Design review of the part built by this model. Coordinates are the model's own, in mm. A direction names the side the tool comes from. Coordinates: 2 decimals unless noted, no trailing zeros. Loops run counter-clockwise (first coordinate to the right, second up) from the corner with the lowest first, then second, coordinate; pieces in that order, holes last.
Q1. For P1, Ø0.5, axis at x = -14, z = 1, coming from the -Y side; P2, Ø0.8, axis at y = -2.5, z = 0.5, coming from the +X side, all flat-tipped, find the tip position at first contact; note any pin that passes through.
Q2. Add section A-A on y = 4. Give the boundary of the cut face in (x, z).
Q3. Machinability: for faces 1 (the face through (1.52, 8.87, 0.78)), 2 (the face through (-12, 4.877, 1)), 3 (the face through (9, 7, 1.588)), which of the approach directions +Z, -Z, +X, -X, +Y, -Y give a long, thin tool a straight path to every point of the face, cutting with its end or side? Answer none if there is none.
Q4. Add section B-B on x = 5.5. Give the boundary of the cut face in (y, z), and give its area (3 significant figures).
Q5. Add section C-C on z = 1.1. Give the number of separate pieces and of enclosed holes in the cut face, and give its area (3 significant figures).
Q6. Draft analysis for pull direction X (two halves, no side actions). For faces 4 (the face through (-13.07, 14, 0.78)), 5 (the face through (10.44, -1.11, 0.78)), 6 (the face through (16.226, 7.464, 0.783)), state which applies: released by +X, released by -X, zero draft, split by the parting line, or undercut.
Q7. Wall thickness on probe 1 along X at (y, z) = (12.5, 1.35); probe 2 along Y at (x, z) = (8.5, 0.3); probe 3 along X at (y, z) = (13, 1.05): over which ranges is each line inside the solid? List them lowest first.
Q8. Add section D-D on y = -15. Give the boundary of the cut face in (x, z).
```python
from build123d import *
from build123d.topology import SkipClean

# Parameters (mm, degrees)
SKETCH1_R           = 1.4224
BOSS_EXTRUDE1_DEPTH = 1.5875
CUT_EXTRUDE3_DEPTH  = 31.574112518
CUT_EXTRUDE4_DEPTH  = 31.574112518
SKETCH4_R           = 1.1049
BOSS_EXTRUDE2_DEPTH = 1.5875
SKETCH4_3_R         = 1.1049
CUT_EXTRUDE5_DEPTH  = 2.54


with BuildPart() as part:
    # Sketch1 → Boss-Extrude1 (new body)
    with BuildSketch(Plane.XY):
        with BuildLine():
            Line((-5.027565338, -0.720652536), (-4.515281158, 3.5306))
            Line((-4.515281158, 3.5306), (-2.860140414, 4.994714494))
            Line((-2.860140414, 4.994714494), (-4.980602482, 7.391837931))
            Line((-4.980602482, 7.391837931), (-2.583479045, 9.5123))
            Line((-2.583479045, 9.5123), (-0.463016976, 7.115176563))
            Line((-0.463016976, 7.115176563), (11.876076152, 18.030166811))
            ThreePointArc((11.876076152, 18.030166811), (-16.886200405, -13.453041882), (20.228041911, 7.546815251))
            Line((20.228041911, 7.546815251), (8.405899773, -2.910887338))
            Line((8.405899773, -2.910887338), (10.526361842, -5.308010776))
            Line((10.526361842, -5.308010776), (8.129238404, -7.428472845))
            Line((8.129238404, -7.428472845), (6.008776335, -5.031349407))
            Line((6.008776335, -5.031349407), (4.353635591, -6.495463901))
            Line((4.353635591, -6.495463901), (1.815981702, -6.489359631))
            Line((1.815981702, -6.489359631), (-5.455454601, -12.9215711))
            Line((-5.455454601, -12.9215711), (-8.720293025, -9.230761998))
            Line((-8.720293025, -9.230761998), (-2.425370717, -3.662361234))
            Line((-2.425370717, -3.662361234), (-5.027565338, -0.720652536))
        make_face()
        with Locations((0, 18.415)):
            Circle(SKETCH1_R, mode=Mode.SUBTRACT)
        with Locations((0, -18.415)):
            Circle(SKETCH1_R, mode=Mode.SUBTRACT)
    extrude(amount=BOSS_EXTRUDE1_DEPTH)

    # Sketch2 → Cut-Extrude3 (cut, through all)
    with BuildSketch(Plane.XY.offset(1.5875)):
        with BuildLine():
            Line((-7.084965338, 4.8768), (-21.031997569, 4.8768))
            ThreePointArc((-21.031997569, 4.8768), (-21.588987692, -0.209070373), (-20.933606898, -5.2832))
            Line((-20.933606898, -5.2832), (-7.084965338, -5.2832))
            Line((-7.084965338, -5.2832), (-7.084965338, 4.8768))
        make_face()
    extrude(amount=-CUT_EXTRUDE3_DEPTH, mode=Mode.SUBTRACT)

    # Sketch3 → Cut-Extrude4 (cut, through all)
    with BuildSketch(Plane(origin=(0, 0, 0), x_dir=(-1, 0, 0), z_dir=(0, 0, -1))):
        with BuildLine():
            Line((-20.871224203, -5.5245), (-16.984058744, -5.5245))
            Line((-16.984058744, -5.5245), (-16.984058744, 4.677232838))
            Line((-16.984058744, 4.677232838), (-20.228041911, 7.546815251))
            ThreePointArc((-20.228041911, 7.546815251), (-21.563910577, 1.061065789), (-20.871224203, -5.5245))
        make_face()
    extrude(amount=-CUT_EXTRUDE4_DEPTH, mode=Mode.SUBTRACT)

    # Sketch4 → Boss-Extrude2 (add)
    # profile 1 of 5: a face of its own
    with BuildSketch(Plane(origin=(0, 0, 0), x_dir=(-1, 0, 0), z_dir=(0, 0, -1))):
        with BuildLine():
            Line((-16.984058744, 5.5245), (-16.984058744, 4.677232838))
            Line((-16.984058744, 4.677232838), (-12.420130291, 0.640045174))
            Line((-12.420130291, 0.640045174), (-3.551213542, 10.666109075))
            Line((-3.551213542, 10.666109075), (-8.959431605, 15.450143591))
            ThreePointArc((-8.959431605, 15.450143591), (-11.076965007, 14.009967805), (-12.966760902, 12.28175327))
            Line((-12.966760902, 12.28175327), (-15.004080987, 13.83506338))
            ThreePointArc((-15.004080987, 13.83506338), (-17.674010029, 13.475162132), (-17.314108781, 10.80523309))
            Line((-17.314108781, 10.80523309), (-15.276788696, 9.25192298))
            ThreePointArc((-15.276788696, 9.25192298), (-16.237733521, 7.437362555), (-16.984058744, 5.5245))
        make_face()
        with Locations((-16.159094884, 12.320148235)):
            Circle(SKETCH4_R, mode=Mode.SUBTRACT)
    # profile 2 of 5: a face of its own
    with BuildSketch(Plane(origin=(0, 0, 0), x_dir=(-1, 0, 0), z_dir=(0, 0, -1))):
        with BuildLine():
            ThreePointArc((-1.288911844, -17.813395463), (-0.402766027, -17.855423019), (0.484373541, -17.853395586))
            Line((0.484373541, -17.853395586), (0.725034865, -19.638742704))
            ThreePointArc((0.725034865, -19.638742704), (0.955229003, -17.361074333), (-1.288911844, -17.813395463))
        make_face()
    # profile 3 of 5: a face of its own
    with BuildSketch(Plane(origin=(0, 0, 0), x_dir=(-1, 0, 0), z_dir=(0, 0, -1))):
        with BuildLine():
            ThreePointArc((4.327227494, -21.151907768), (2.884204284, -21.396482553), (1.427926458, -21.542727915))
            ThreePointArc((1.427926458, -21.542727915), (2.969033821, -22.025790864), (4.327227494, -21.151907768))
        make_face()
    # profile 4 of 5: a face of its own
    with BuildSketch(Plane(origin=(0, 0, 0), x_dir=(-1, 0, 0), z_dir=(0, 0, -1))):
        with BuildLine():
            ThreePointArc((1.288911844, 17.813395463), (0, 17.859965052), (-1.288911844, 17.813395463))
            ThreePointArc((-1.288911844, 17.813395463), (0, 16.9926), (1.288911844, 17.813395463))
        make_face()
    # profile 5 of 5: a face of its own
    with BuildSketch(Plane(origin=(0, 0, 0), x_dir=(-1, 0, 0), z_dir=(0, 0, -1))):
        with BuildLine():
            ThreePointArc((14.223312513, 16.242705475), (13.475162132, 17.674010029), (11.896845513, 18.016469323))
            ThreePointArc((11.896845513, 18.016469323), (13.0901575, 17.169038314), (14.223312513, 16.242705475))
        make_face()
    extrude(amount=-BOSS_EXTRUDE2_DEPTH)

    # Sketch4<3> → Cut-Extrude5 (cut)
    with SkipClean():  # the faces are left unmerged after this step: merging them gives an invalid solid
        with BuildSketch(Plane(origin=(0, 0, 0), x_dir=(-1, 0, 0), z_dir=(0, 0, -1))):
            with BuildLine():
                ThreePointArc((-20.871224203, -5.5245), (-12.595886757, -17.534872021), (1.427926458, -21.542727915))
                ThreePointArc((1.427926458, -21.542727915), (1.026270462, -21.020335978), (0.826620277, -20.392354546))
                Line((0.826620277, -20.392354546), (0.725034865, -19.638742704))
                ThreePointArc((0.725034865, -19.638742704), (-0.955229003, -19.468925667), (-1.288911844, -17.813395463))
                ThreePointArc((-1.288911844, -17.813395463), (-11.010431484, -14.062316673), (-16.984058744, -5.5245))
                Line((-16.984058744, -5.5245), (-20.871224203, -5.5245))
            make_face()
            with BuildLine():
                ThreePointArc((4.602470139, -19.883377319), (4.576225926, -20.541808877), (4.327227494, -21.151907768))
                ThreePointArc((4.327227494, -21.151907768), (14.915810742, -15.609186074), (20.933606898, -5.2832))
                Line((20.933606898, -5.2832), (17.060660873, -5.2832))
                ThreePointArc((17.060660873, -5.2832), (12.247990597, -12.998656777), (4.260223404, -17.344418359))
                Line((4.260223404, -17.344418359), (4.602470139, -19.883377319))
            make_face()
            with BuildLine():
                Line((-11.876076152, 18.030166811), (-8.959431605, 15.450143591))
                ThreePointArc((-8.959431605, 15.450143591), (-5.258647708, 17.068244665), (-1.288911844, 17.813395463))
                ThreePointArc((-1.288911844, 17.813395463), (0, 19.8374), (1.288911844, 17.813395463))
                ThreePointArc((1.288911844, 17.813395463), (5.420875683, 17.017416329), (9.25192298, 15.276788696))
                Line((9.25192298, 15.276788696), (10.80523309, 17.314108781))
                ThreePointArc((10.80523309, 17.314108781), (11.28937197, 17.76113274), (11.896845513, 18.016469323))
                ThreePointArc((11.896845513, 18.016469323), (0.01243973, 21.589996416), (-11.876076152, 18.030166811))
            make_face()
            with BuildLine():
                Line((13.83506338, 15.004080987), (12.28175327, 12.966760902))
                ThreePointArc((12.28175327, 12.966760902), (15.276744775, 9.251995502), (17.181244816, 4.8768))
                Line((17.181244816, 4.8768), (21.031997569, 4.8768))
                ThreePointArc((21.031997569, 4.8768), (18.521073783, 11.09495047), (14.223312513, 16.242705475))
                ThreePointArc((14.223312513, 16.242705475), (14.13793931, 15.589304916), (13.83506338, 15.004080987))
            make_face()
            with Locations((12.320148235, 16.159094884)):
                Circle(SKETCH4_3_R)
            with Locations((2.714545208, -20.137865932)):
                Circle(SKETCH4_3_R)
        extrude(amount=-CUT_EXTRUDE5_DEPTH, mode=Mode.SUBTRACT)


solid = part.part
```
Entries:
1. P1: stops at y = -11.4
1. P2: stops at x = 16.98
2. outline: (-7.08, 0) - (-3.98, 0) - (-3.98, 1.59) - (-7.08, 1.59) - close; (9.45, 0) - (16.98, 0) - (16.98, 1.59) - (9.45, 1.59) - close
3. face 1: +Z, -Z
3. face 2: +Z, -Z, -X
3. face 3: +Z, +X, -X, +Y, -Y
4. outline: (-16.99, 0) - (-5.48, 0) - (-5.48, 1.59) - (-16.99, 1.59) - close; (8.46, 0) - (16.99, 0) - (16.99, 1.59) - (8.46, 1.59) - close
4. area: 31.8 mm2
5. separate pieces: 1
5. enclosed holes: 4
5. area: 682 mm2
6. face 4: released by -X
6. face 5: undercut
6. face 6: released by +X
7. probe 1: x = -12.76 to 12.76, 13.25 to 15.07, 17.25 to 18.06
7. probe 2: y = -15.71 to -7.1, -3.02 to -2.83, 5.07 to 15.71
7. probe 3: x = -12.31 to 12.25, 13.91 to 15.29, 17.03 to 17.94
8. outline: (-9.69, 0) - (9.69, 0) - (9.69, 1.59) - (-9.69, 1.59) - close
